Check sheet for the modelled part. Datum: model origin and axes. Units: mm. Coordinates: 2 decimals unless noted, no trailing zeros. Loops run counter-clockwise (first coordinate to the right, second up) from the corner with the lowest first, then second, coordinate; pieces in that order, holes last. Notation, with made-up numbers: M -36.5,6.25 L -17.5,6.25 A18 cw -17.5,21.25 Z; hole C 72.25,-3 d9. An arc over 180 degrees is marked long. Use CSV: the item, a comma, the result in double quotes. Start each with the question number.
(1) Section check C-C on x = 94. Record the cut outline in (y, z), and give its area (4 significant figures).
(2) Scan lines: line 1 (Z direction, x = -37, y = 0); line 2 (Z direction, x = -76.5, y = -2.5); line 3 (Y direction, x = -177, z = -0.5). Record each from-to range of solid material in increasing order.
(3) Draft check along X on faces 1 (the flat face through (-210, -40, -13)), 2 (the flat face through (178.5, 0, 42)), 3 (the cylindrical face through (-2.94, -9.041, -40.715)). Enter one of: pulls with the +X half, pulls with the -X half, needs draft (parallel to the pull), parting line crosses it, or undercut.
(4) Section check B-B on z = 0. Record the cut outline in (x, y), and give its area (3 significant figures).
(5) Go/stop test with flat-tipped pins: pin 1 Ø5 at (x, y) = (-57, -21.5) entering from +Z; pin 2 Ø5 at (x, y) = (109.5, -5.5) entering from +Z; pin 3 Ø3 at (x, y) = (-140, 18) entering from +Z. Record where each tip stops, or that it passes through.
(6) Section check D-D on z = 33. Record the cut outline in (x, y).
(7) Section check A-A on y = 0. Record the cut outline in (x, z), and give its area (3 significant figures).
from build123d import *

# Parameters (mm, degrees)
SKETCH12_R              = 44.45
SKETCH12_R_2            = 41.7068
PIPE_0_5_SCH_40_1_DEPTH = 420
CUT_EXTRUDE1_DEPTH      = 50
CUT_EXTRUDE1_DEPTH_BACK = 50
SKETCH13_W              = 37
SKETCH13_H              = 75


with BuildPart() as part:
    # Sketch12 → Pipe 0.5 SCH 40(1) (new body)
    with BuildSketch(Plane.YZ.offset(-210)):
        Circle(SKETCH12_R)
        Circle(SKETCH12_R_2, mode=Mode.SUBTRACT)
    extrude(amount=PIPE_0_5_SCH_40_1_DEPTH)

    # Sketch13 → Cut-Extrude1 (cut, two sides: drawn at the far end of the back side and taken through both)
    with BuildSketch(Plane.XY.offset(-CUT_EXTRUDE1_DEPTH_BACK)):
        with Locations((160, 0)):
            Rectangle(SKETCH13_W, SKETCH13_H)
    extrude(amount=CUT_EXTRUDE1_DEPTH + CUT_EXTRUDE1_DEPTH_BACK, mode=Mode.SUBTRACT)


solid = part.part
Outcome:
1,outline,"C 0,0 d88.9; hole C 0,0 d83.41"
1,area,"742.5 mm²"
2,line 1,"z = -44.45 to -41.71, 41.71 to 44.45"
2,line 2,"z = -44.38 to -41.63, 41.63 to 44.38"
2,line 3,"y = -44.45 to -41.7, 41.7 to 44.45"
3,face 1,"pulls with the -X half"
3,face 2,"undercut"
3,face 3,"needs draft"
4,outline,"M -210,-44.45 L 210,-44.45 L 210,-41.71 L -210,-41.71 Z; M -210,41.71 L 210,41.71 L 210,44.45 L -210,44.45 Z"
4,area,"2,300 mm²"
5,pin 1,"stops at z = 40.18"
5,pin 2,"stops at z = 44.35"
5,pin 3,"stops at z = 41.27"
6,outline,"M -210,-29.78 L 141.5,-29.78 L 141.5,-25.5 L -210,-25.5 Z; M -210,25.5 L 141.5,25.5 L 141.5,29.78 L -210,29.78 Z; M 178.5,-29.78 L 210,-29.78 L 210,-25.5 L 178.5,-25.5 Z; M 178.5,25.5 L 210,25.5 L 210,29.78 L 178.5,29.78 Z"
7,outline,"M -210,-44.45 L 141.5,-44.45 L 141.5,-41.71 L -210,-41.71 Z; M -210,41.71 L 141.5,41.71 L 141.5,44.45 L -210,44.45 Z; M 178.5,-44.45 L 210,-44.45 L 210,-41.71 L 178.5,-41.71 Z; M 178.5,41.71 L 210,41.71 L 210,44.45 L 178.5,44.45 Z"
7,area,"2,100 mm²"
